Work out the finished part from the listing and answer in its coordinate system (mm). Coordinates: 2 decimals unless noted, no trailing zeros. Order: outer loops, then holes, each group sorted by start corner. A loop starts at its lowest first (then second) coordinate and runs counter-clockwise, first axis right, second up. Notation, with made-up numbers: (89, -2.5) -> (148, -2.5) arc R24 ccw to (148, 21.5) -> close; hole circle Ø3 at (85.25, -38.5). An arc over 180 degrees is marked (long way). Use one line per item in the form item = value.
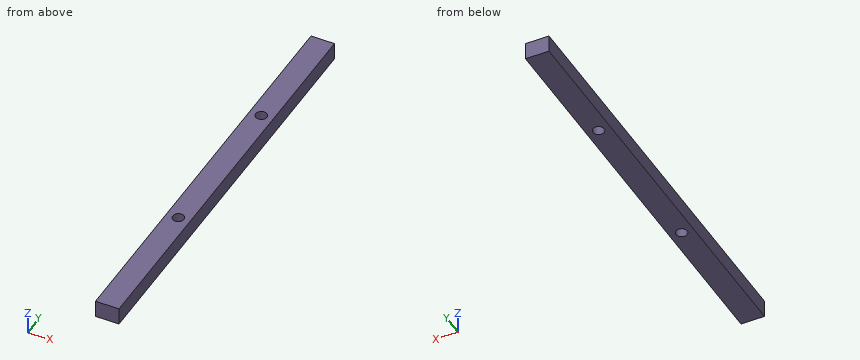
Solid Edge part; units mm, degrees
sketch "Sketch1" plane through (0, 0, 0) normal (0, 0, 1) x (1, 0, 0)
  circle A0 centre (3.81, 29.9081) radius 1.2192
  circle A1 centre (3.81, 64.8331) radius 1.2192
  line L0 (6.334, 90.6845) -> (6.334, 0)
  line L1 (6.334, 0) -> (1.254, 0)
  line L2 (1.254, 0) -> (1.254, 90.6845)
  line L3 (1.254, 90.6845) -> (6.334, 90.6845)
extrude "Protrusion1" add sketch "Sketch1" along normal up to vertex (3.75 mm away)
(1) Section B-B on z = 2.15 is taken. Write down the section's boundary in (x, y), plus the area to 3 significant figures.
Data:
outline = (1.25, 0) -> (6.33, 0) -> (6.33, 90.68) -> (1.25, 90.68) -> close; hole circle Ø2.44 at (3.81, 29.91); hole circle Ø2.44 at (3.81, 64.83)
area = 451 mm²
(2) Straight lines are drawn through the part: line 1 along Y through (x, z) = (3.81, 1.8); line 2 along Y through (x, z) = (3.9, 2.2). For each, find the intervals that lie inside material, in ascending order.
Data:
line_1 = 0 to 28.69, 31.13 to 63.61, 66.05 to 90.68
line_2 = 0 to 28.69, 31.12 to 63.62, 66.05 to 90.68
(3) Section A-A on x = 3.81 is taken. Write down the section's boundary in (y, z), plus the area to 3 significant figures.
Data:
outline = (0, 0) -> (28.69, 0) -> (28.69, 3.75) -> (0, 3.75) -> close; (31.13, 0) -> (63.61, 0) -> (63.61, 3.75) -> (31.13, 3.75) -> close; (66.05, 0) -> (90.68, 0) -> (90.68, 3.75) -> (66.05, 3.75) -> close
area = 322 mm²
